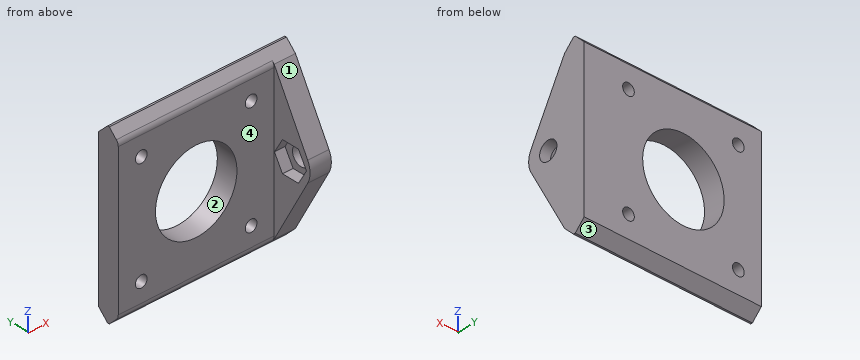
from build123d import *

# Parameters (mm, degrees)
SKETCH1_W           = 44
SKETCH1_H           = 49
SKETCH1_R           = 11.5
SKETCH1_R_2         = 1.65
BOSS_EXTRUDE1_DEPTH = 6
CHAMFER1_SIZE       = 2.75
BOSS_EXTRUDE2_DEPTH = 3
SKETCH3_R           = 2.65
BOSS_EXTRUDE3_DEPTH = 3
BOSS_EXTRUDE4_DEPTH = 6
FILLET1_R           = 2


with BuildPart() as part:
    # Sketch1 → Boss-Extrude1 (new body)
    with BuildSketch(Plane(origin=(0, 0, 0), x_dir=(1, 0, 0), z_dir=(0, 1, 0))):
        Rectangle(SKETCH1_W, SKETCH1_H)
        with Locations(Location((0, 0, 0), (0, 0, 270))):
            Circle(SKETCH1_R, mode=Mode.SUBTRACT)
        with Locations(Location((15.5, 15.5, 0), (0, 0, 270))):
            Circle(SKETCH1_R_2, mode=Mode.SUBTRACT)
        with Locations(Location((15.5, -15.5, 0), (0, 0, 270))):
            Circle(SKETCH1_R_2, mode=Mode.SUBTRACT)
        with Locations(Location((-15.5, -15.5, 0), (0, 0, 270))):
            Circle(SKETCH1_R_2, mode=Mode.SUBTRACT)
        with Locations(Location((-15.5, 15.5, 0), (0, 0, 270))):
            Circle(SKETCH1_R_2, mode=Mode.SUBTRACT)
    extrude(amount=BOSS_EXTRUDE1_DEPTH)

    # Chamfer1
    chamfer1_edges = [part.edges().sort_by_distance(p)[0] for p in [
        (0, 6, 24.5),
        (0, 0, 24.5),
        (0, 0, -24.5),
        (0, 6, -24.5),
    ]]
    chamfer(chamfer1_edges, length=CHAMFER1_SIZE)

    # Sketch2 → Boss-Extrude2 (add)
    with BuildSketch(Plane(origin=(22, 0, 0), x_dir=(0, 0, -1), z_dir=(1, 0, 0))):
        with BuildLine():
            Line((-21.75, 6), (21.75, 6))
            Line((21.75, 6), (21.75, 0))
            Line((21.75, 0), (2.866847379, -10.270786099))
            ThreePointArc((2.866847379, -10.270786099), (0, -11), (-2.866847379, -10.270786099))
            Line((-2.866847379, -10.270786099), (-21.75, 0))
            Line((-21.75, 0), (-21.75, 6))
        make_face()
        Polygon((0, -9.907477288), (4.25, -7.453738644), (4.25, -2.546261356), (0, -0.092522712), (-4.25, -2.546261356), (-4.25, -7.453738644), align=None, mode=Mode.SUBTRACT)
    extrude(amount=BOSS_EXTRUDE2_DEPTH)

    # Sketch3 → Boss-Extrude3 (add)
    # profile 1 of 2: a face of its own
    with BuildSketch(Plane(origin=(25, 0, 0), x_dir=(0, 0, -1), z_dir=(1, 0, 0))):
        with BuildLine():
            Line((21.75, 6), (-21.75, 6))
            Line((-21.75, 6), (-21.75, 0))
            Line((-21.75, 0), (-2.866847379, -10.270786099))
            ThreePointArc((-2.866847379, -10.270786099), (0, -11), (2.866847379, -10.270786099))
            Line((2.866847379, -10.270786099), (21.75, 0))
            Line((21.75, 0), (21.75, 6))
        make_face()
        Polygon((4.25, -2.546261356), (4.25, -7.453738644), (0, -9.907477288), (-4.25, -7.453738644), (-4.25, -2.546261356), (0, -0.092522712), align=None, mode=Mode.SUBTRACT)
    # profile 2 of 2: a face of its own
    with BuildSketch(Plane(origin=(25, 0, 0), x_dir=(0, 0, -1), z_dir=(1, 0, 0))):
        Polygon((4.25, -7.453738644), (0, -9.907477288), (-4.25, -7.453738644), (-4.25, -2.546261356), (0, -0.092522712), (4.25, -2.546261356), align=None)
        with Locations((0, -5)):
            Circle(SKETCH3_R, mode=Mode.SUBTRACT)
    extrude(amount=BOSS_EXTRUDE3_DEPTH)

    # Sketch4 → Boss-Extrude4 (add)
    with BuildSketch(Plane(origin=(22, 0, 0), x_dir=(0, 0, -1), z_dir=(1, 0, 0))):
        Polygon((-21.75, 0), (-21.75, 6), (-24.5, 3.25), (-24.5, 2.75), align=None)
        Polygon((21.75, 6), (21.75, 0), (24.5, 2.75), (24.5, 3.25), align=None)
    extrude(amount=BOSS_EXTRUDE4_DEPTH)

    # Fillet1
    fillet1_edges = [part.edges().sort_by_distance(p)[0] for p in [
        (0, 0, 21.75),
        (0, 0, -21.75),
    ]]
    fillet(fillet1_edges, radius=FILLET1_R)


solid = part.part
Here's how the part is built. I have some questions about the finished solid (model axes, mm). Face numbers are marked on the shaded views. Coordinates: 2 decimals unless noted, no trailing zeros. Order: outer loops, then holes, each group sorted by start corner. A loop starts at its lowest first (then second) coordinate and runs counter-clockwise, first axis right, second up. Notation, with made-up numbers: M -8.5,37.25 L 48.5,37.25 A26 cw 48.5,56.25 Z; hole C -5,-38.75 d5. An arc over 180 degrees is marked long. Answer as CSV lines item,"result".
Item 1: For pin 1 (2 mm diameter, centred on y = -4, z = 17.5, fed in from -X); pin 2 (8 mm diameter, centred on y = -5.5, z = -19, fed in from -X); pin 3 (1.5 mm diameter, centred on x = 23.5, y = -4, fed in from -Z); pin 4 (1.5 mm diameter, centred on x = 18.5, z = 17, fed in from -Y), each with a flat end and sliding along its axis, tell me the tip position at first contact or that it passes through.
Results found:
pin 1,"through"
pin 2,"x = 22"
pin 3,"z = -15.77"
pin 4,"y = 0"
Item 2: Imagine slicing it at D-D on z = -15.5. Write out the boundary of the cut face in (x, y), plus the area to 3 significant figures.
Results found:
outline,"M -22,0 L -17.15,0 L -17.15,6 L -22,6 Z; M -13.85,0 L 13.85,0 L 13.85,6 L -13.85,6 Z; M 17.15,0 L 22,0 L 22,-3.4 L 28,-3.4 L 28,6 L 17.15,6 Z"
area,"281 mm2"
Item 3: Imagine slicing it at A-A on x = 15.5. Write out the boundary of the cut face in (y, z).
Results found:
outline,"M 0,-20.92 A2 ccw 0.59,-22.34 L 2.75,-24.5 L 3.25,-24.5 L 6,-21.75 L 6,-17.15 L 0,-17.15 Z; M 0,-13.85 L 6,-13.85 L 6,13.85 L 0,13.85 Z; M 0,17.15 L 6,17.15 L 6,21.75 L 3.25,24.5 L 2.75,24.5 L 0.59,22.34 A2 ccw 0,20.92 Z"
Item 4: If I drill on line 1 (X direction, y = 1.9, z = 15.5); line 2 (Y direction, x = 26, z = 0); line 3 (X direction, y = 2.9, z = 0), over which ranges is the centre line in solid material (lowest first)?
Results found:
line 1,"-22 to -17.15, -13.85 to 13.85, 17.15 to 28"
line 2,"-11 to -7.65, -2.35 to 6"
line 3,"-22 to -11.5, 11.5 to 28"
Item 5: Imagine slicing it at B-B on y = 4. Write out the boundary of the cut face in (x, z).
Results found:
outline,"M -22,-23.75 L 28,-23.75 L 28,23.75 L -22,23.75 Z; hole C -15.5,-15.5 d3.3; hole C -15.5,15.5 d3.3; hole C 0,0 d23; hole C 15.5,-15.5 d3.3; hole C 15.5,15.5 d3.3"
Item 6: Imagine slicing it at C-C on x = 0. Write out the boundary of the cut face in (y, z), plus the area to 3 significant figures.
Results found:
outline,"M 0,-20.92 A2 ccw 0.59,-22.34 L 2.75,-24.5 L 3.25,-24.5 L 6,-21.75 L 6,-11.5 L 0,-11.5 Z; M 0,11.5 L 6,11.5 L 6,21.75 L 3.25,24.5 L 2.75,24.5 L 0.59,22.34 A2 ccw 0,20.92 Z"
area,"141 mm2"
Item 7: We'd pull the mould along Z, two halves only. Please class the marked faces 1, 2, 3 and 4: +Z half, -Z half, draft (parallel to the pull), parting line (faces both ways), or undercut.
Results found:
face 1,"+Z half"
face 2,"undercut"
face 3,"-Z half"
face 4,"draft"
